Could you check a few things on this model? Use its own coordinates, in mm. Face numbers are marked on the shaded views. A direction names the side the tool comes from. Round coordinates to 2 decimals unless told otherwise and drop trailing zeros. Write each loop counter-clockwise with the first axis right and the second up, starting at its lowest first coordinate (ties: lowest second). Pieces come first, ordered by that corner, then holes. Notation, with made-up numbers: (46, -6.75) -> (92, -6.75) arc R23 ccw to (92, 10.25) -> close; hole circle Ø10 at (43.25, 70). An arc over 180 degrees is marked (long way). Return JSON: item names as keys, results as strings.
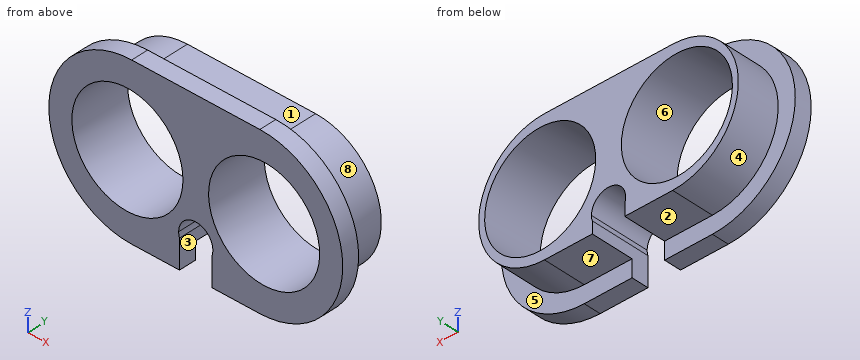
from build123d import *

# Parameters (mm, degrees)
EXTRUDE_1_DEPTH     = 2
EXTRUDE_2_DEPTH     = 5
CUT_EXTRUDE_1_REACH = 22.951
SKETCH_3_R          = 6.5


with BuildPart() as part:
    # 草圖2 → 填料-伸長1 (new body)
    with BuildSketch(Plane(origin=(0, 0, 0), x_dir=(1, 0, 0), z_dir=(0, 1, 0))):
        with BuildLine():
            Line((-7.5, 9.7), (7.5, 9.7))
            ThreePointArc((7.5, 9.7), (17.2, 0), (7.5, -9.7))
            Line((7.5, -9.7), (-7.5, -9.7))
            ThreePointArc((-7.5, -9.7), (-17.2, 0), (-7.5, 9.7))
        make_face()
    extrude(amount=-EXTRUDE_1_DEPTH)

    # 草圖1 → 填料-伸長2 (add)
    with BuildSketch(Plane(origin=(0, 0, 0), x_dir=(1, 0, 0), z_dir=(0, 1, 0))):
        with BuildLine():
            Line((-7.5, 7.7), (7.5, 7.7))
            ThreePointArc((7.5, 7.7), (15.2, 0), (7.5, -7.7))
            Line((7.5, -7.7), (-7.5, -7.7))
            ThreePointArc((-7.5, -7.7), (-15.2, 0), (-7.5, 7.7))
        make_face()
    extrude(amount=EXTRUDE_2_DEPTH)

    # 草圖3 → 除料-伸長1 (cut, up to next)
    with BuildSketch(Plane.XZ.offset(2), mode=Mode.PRIVATE) as cut_extrude_1_sk1:
        with Locations(Location((-8, 0, 0), (0, 0, 270))):
            Circle(SKETCH_3_R)
    cut_extrude_1_tool1 = extrude(cut_extrude_1_sk1.sketch, amount=-CUT_EXTRUDE_1_REACH, mode=Mode.PRIVATE) & part.part
    # 草圖3 → 除料-伸長1 (cut, up to next)
    with BuildSketch(Plane.XZ.offset(2), mode=Mode.PRIVATE) as cut_extrude_1_sk2:
        with Locations(Location((8, 0, 0), (0, 0, 270))):
            Circle(SKETCH_3_R)
    cut_extrude_1_tool2 = extrude(cut_extrude_1_sk2.sketch, amount=-CUT_EXTRUDE_1_REACH, mode=Mode.PRIVATE) & part.part
    # 草圖3 → 除料-伸長1 (cut, up to next)
    with BuildSketch(Plane.XZ.offset(2), mode=Mode.PRIVATE) as cut_extrude_1_sk3:
        with BuildLine():
            ThreePointArc((2, -5.7), (0, -3.7), (-2, -5.7))
            Line((-2, -5.7), (2, -5.7))
        make_face()
    cut_extrude_1_tool3 = extrude(cut_extrude_1_sk3.sketch, amount=-CUT_EXTRUDE_1_REACH, mode=Mode.PRIVATE) & part.part
    # 草圖3 → 除料-伸長1 (cut, up to next)
    with BuildSketch(Plane.XZ.offset(2), mode=Mode.PRIVATE) as cut_extrude_1_sk4:
        with BuildLine():
            Line((2, -5.7), (-2, -5.7))
            ThreePointArc((-2, -5.7), (-1.974841766, -6.016227766), (-1.9, -6.3244998))
            Line((-1.9, -6.3244998), (-1.9, -9.7))
            Line((-1.9, -9.7), (1.9, -9.7))
            Line((1.9, -9.7), (1.9, -6.3244998))
            ThreePointArc((1.9, -6.3244998), (1.974841766, -6.016227766), (2, -5.7))
        make_face()
    cut_extrude_1_tool4 = extrude(cut_extrude_1_sk4.sketch, amount=-CUT_EXTRUDE_1_REACH, mode=Mode.PRIVATE) & part.part
    add(cut_extrude_1_tool1.solids().sort_by_distance((-8, -2, 0))[0], mode=Mode.SUBTRACT)
    add(cut_extrude_1_tool2.solids().sort_by_distance((8, -2, 0))[0], mode=Mode.SUBTRACT)
    add(cut_extrude_1_tool3.solids().sort_by_distance((0, -2, -4.851174))[0], mode=Mode.SUBTRACT)
    add(cut_extrude_1_tool4.solids().sort_by_distance((0, -2, -7.690335))[0], mode=Mode.SUBTRACT)


solid = part.part
1) I want a section at A-A, the plane z = 0. Please give me the cut outline in (x, y), and give its area (3 significant figures).
Return value:
{"outline": "(-17.2, -2) -> (-14.5, -2) -> (-14.5, 5) -> (-15.2, 5) -> (-15.2, 0) -> (-17.2, 0) -> close; (-1.5, -2) -> (1.5, -2) -> (1.5, 5) -> (-1.5, 5) -> close; (14.5, -2) -> (17.2, -2) -> (17.2, 0) -> (15.2, 0) -> (15.2, 5) -> (14.5, 5) -> close", "area": "38.8 mm²"}
2) I want a section at C-C, the plane x = 8. Please give me the cut outline in (y, z), and give its area (3 significant figures).
Return value:
{"outline": "(-2, -9.69) -> (0, -9.69) -> (0, -7.68) -> (5, -7.68) -> (5, -6.5) -> (-2, -6.5) -> close; (-2, 6.5) -> (5, 6.5) -> (5, 7.68) -> (0, 7.68) -> (0, 9.69) -> (-2, 9.69) -> close", "area": "24.6 mm²"}
3) Will these pins go through, and if not, where does the flat tip stop? pin 1 Ø5 at (x, z) = (3.5, -1.5) entering from +Y; pin 2 Ø1.5 at (x, y) = (13.5, 3) entering from -Z; pin 3 Ø1 at (x, y) = (13.5, 3) entering from +Z; pin 4 Ø3 at (x, y) = (3, 3) entering from +Z.
Return value:
{"pin 1": "y = 5", "pin 2": "z = -5.63", "pin 3": "z = 5.39", "pin 4": "z = 7.7"}
4) For the marked faces 1, 2, 3, 4 and 5, which set-ups out of +Z, -Z, +X, -X, +Y, -Y let a thin tool reach every point of the face, with its end or its side?
Return value:
{"face 1": "+Z, +X, -X, +Y", "face 2": "-Z, +X, -X, +Y", "face 3": "-Z, +Y, -Y", "face 4": "-X, +Y", "face 5": "+Y"}
5) If I drill on probe 1 along X at (y, z) = (0.25, 0); probe 2 along X at (y, z) = (1.5, -2); probe 3 along Z at (x, y) = (14, -1.25), over which ranges is the centre line in solid material (lowest first)? Write a range as [from, to].
Return value:
{"probe 1": "[-15.2, -14.5], [-1.5, 1.5], [14.5, 15.2]", "probe 2": "[-14.94, -14.18], [-1.82, 1.82], [14.18, 14.94]", "probe 3": "[-7.2, -2.5], [2.5, 7.2]"}
6) Thinking about a two-plate mould opening in X: for the marked faces 6, 7 and 8, which applies, pulls with the +X half, pulls with the -X half, needs draft (parallel to the pull), parting line crosses it, or undercut?
Return value:
{"face 6": "undercut", "face 7": "needs draft", "face 8": "pulls with the +X half"}
7) I want a section at B-B, the plane y = -1.5. Please give me the cut outline in (x, z), and give its area (3 significant figures).
Return value:
{"outline": "(-7.5, -9.7) -> (-1.9, -9.7) -> (-1.9, -6.32) arc R2 cw (long way) to (1.9, -6.32) -> (1.9, -9.7) -> (7.5, -9.7) arc R9.7 ccw to (7.5, 9.7) -> (-7.5, 9.7) arc R9.7 ccw to start; hole circle Ø13 at (-8, 0); hole circle Ø13 at (8, 0)", "area": "300 mm²"}
8) I want a section at D-D, the plane z = -8.25. Please give me the cut outline in (x, y).
Return value:
{"outline": "(-12.6, -2) -> (-1.9, -2) -> (-1.9, 0) -> (-12.6, 0) -> close; (1.9, -2) -> (12.6, -2) -> (12.6, 0) -> (1.9, 0) -> close"}
